from build123d import *

# Parameters (mm, degrees)
BOSS_EXTRUDE1_DEPTH     = 9
SKETCH2_R               = 2.25
CUT_EXTRUDE1_DEPTH      = 16.5
SKETCH2_3_R             = 3.75
SKETCH2_3_R_2           = 2.25
CUT_EXTRUDE2_DEPTH      = 1
SKETCH3_R               = 3
BOSS_EXTRUDE2_DEPTH     = 12
CUT_EXTRUDE3_DEPTH      = 26.24364859
CUT_EXTRUDE3_DEPTH_BACK = 26.24364859
SKETCH4_R               = 1


with BuildPart() as part:
    # Sketch1 → Boss-Extrude1 (new body)
    with BuildSketch(Plane.XY):
        Polygon((0, 0), (17.616685226, 9.5), (27.6, 9.5), (27.6, 14.5), (35.6, 14.5), (35.6, 16.5), (26.6, 16.5), (19.116685226, 11.5), (18.116685226, 11.5), (13.116685226, 17.5), (11.616685226, 17.5), (0, 0.25), align=None)
    extrude(amount=BOSS_EXTRUDE1_DEPTH)

    # Sketch2 → Cut-Extrude1 (cut)
    with BuildSketch(Plane(origin=(0, 16.5, 0), x_dir=(1, 0, 0), z_dir=(0, 1, 0))):
        with Locations(Location((31.6, -4.5, 0), (0, 0, 270))):
            Circle(SKETCH2_R)
        Polygon((0, 0), (0, -4), (8.616685226, 0), align=None)
        Polygon((0, -5), (8.616685226, -9), (0, -9), align=None)
    extrude(amount=-CUT_EXTRUDE1_DEPTH, mode=Mode.SUBTRACT)

    # Sketch2<3> → Cut-Extrude2 (cut)
    with BuildSketch(Plane(origin=(0, 16.5, 0), x_dir=(1, 0, 0), z_dir=(0, 1, 0))):
        with Locations(Location((31.6, -4.5, 0), (0, 0, 270))):
            Circle(SKETCH2_3_R)
        with Locations(Location((31.6, -4.5, 0), (0, 0, 270))):
            Circle(SKETCH2_3_R_2, mode=Mode.SUBTRACT)
    extrude(amount=-CUT_EXTRUDE2_DEPTH, mode=Mode.SUBTRACT)

    # Sketch3 → Boss-Extrude2 (add)
    with BuildSketch(Plane(origin=(16.347551937, 13.622959947, 0), x_dir=(0, 0, -1), z_dir=(0.768221279597376, 0.6401843996644799, 0))):
        with Locations(Location((-4.5, 1.046775136, 0), (0, 0, 270))):
            Circle(SKETCH3_R)
    extrude(amount=BOSS_EXTRUDE2_DEPTH)

    # Sketch4 → Cut-Extrude3 (cut, two sides: drawn at the far end of the back side and taken through both)
    with BuildSketch(Plane(origin=(16.347551937, 13.622959947, 0), x_dir=(0, 0, -1), z_dir=(0.768221279597376, 0.6401843996644799, 0)).offset(-CUT_EXTRUDE3_DEPTH_BACK)):
        with Locations(Location((-5.75, 0.046775136, 0), (0, 0, 90))):
            Circle(SKETCH4_R)
        with Locations(Location((-3.25, 0.046775136, 0), (0, 0, 90))):
            Circle(SKETCH4_R)
    extrude(amount=CUT_EXTRUDE3_DEPTH + CUT_EXTRUDE3_DEPTH_BACK, mode=Mode.SUBTRACT)


solid = part.part
Can you work these out from the model? Positions are in its coordinate system, mm. A direction names the side the tool comes from. Coordinates: 2 decimals unless noted, no trailing zeros. Loops run counter-clockwise (first coordinate to the right, second up) from the corner with the lowest first, then second, coordinate; pieces in that order, holes last. Notation, with made-up numbers: M 50,16.25 L 64,16.25 A19 ccw 64,45.25 Z; hole C 72.5,-4 d2. An arc over 180 degrees is marked long. Answer as CSV lines item,"result". Start each with the question number.
1. Suppose I cut it at B-B, the plane y = 7.75. Count the separate pieces of the cut face and the enclosed holes in it, plus the area to 3 significant figures.
2. If I drill on probe 1 along X at (y, z) = (13.75, 4); probe 2 along Y at (x, z) = (28, 7); probe 3 along Y at (x, z) = (18.5, 3.75), over which ranges is the centre line in solid material (lowest first)? Write a range as [from, to].
3. For faces 4 (the face through (24.87, 22.14, 4.46)), 5 (the face through (31, 14.5, 2)), 6 (the face through (29, 15.5, 4)), 7 (the face through (15.1, 15.12, 1.44)), which set-ups out of +Z, -Z, +X, -X, +Y, -Y let a thin tool reach every point of the face, with its end or its side?
4. Thinking about a two-plate mould opening in Y: for faces 1 (the face through (22.911, 14.035, 4.437)), 2 (the face through (12, 17.5, 4)), 3 (the face through (23, 9.5, 4)), which applies, +Y half, -Y half, draft (parallel to the pull), parting line (faces both ways), or undercut?
5. For pin 1 Ø0.5 at (x, z) = (18.5, 6) entering from +Y; pin 2 Ø4 at (x, z) = (30, 6.5) entering from +Y; pin 3 Ø5 at (x, z) = (5, 3.5) entering from +Y, each with a flat end and sliding along its axis, tell me the tip position at first contact or that it passes through.
6. Suppose I cut it at A-A, the plane x = 31.6. List the corners of the cut face in (y, z) for me.
Output:
1,separate pieces,"1"
1,enclosed holes,"2"
1,area,"68.2 mm^2"
2,probe 1,"x = [9.09, 15.39], [17.46, 19.49], [22.48, 27.6]"
2,probe 2,"y = [14.5, 16.5]"
2,probe 3,"y = [9.5, 11.5], [13, 14.35], [16.6, 20.56]"
3,face 4,"+Z, -Z, +X, +Y"
3,face 5,"+Z, -Z, +X, -Y"
3,face 6,"+Y"
3,face 7,"none"
4,face 1,"undercut"
4,face 2,"+Y half"
4,face 3,"-Y half"
5,pin 1,"stops at y = 20.43"
5,pin 2,"stops at y = 16.5"
5,pin 3,"stops at y = 11.39"
6,outline,"M 14.5,0 L 16.5,0 L 16.5,0.75 L 15.5,0.75 L 15.5,2.25 L 14.5,2.25 Z; M 14.5,6.75 L 15.5,6.75 L 15.5,8.25 L 16.5,8.25 L 16.5,9 L 14.5,9 Z"
